The model under review builds one solid part; all positions refer to its coordinate system, in mm. Face numbers are marked on the shaded views. A direction names the side the tool comes from. Give positions to 0.01 mm unless a question says otherwise; leave off trailing zeros. Order: outer loops, then holes, each group sorted by start corner. A loop starts at its lowest first (then second) coordinate and runs counter-clockwise, first axis right, second up. Notation, with made-up numbers: (13.5, 31) -> (52.5, 31) arc R20 cw to (52.5, 35) -> close; hole circle Ø5 at (32, 71). An arc over 180 degrees is marked (long way). Answer as a JSON object with one key per item and string values. Group by question number.
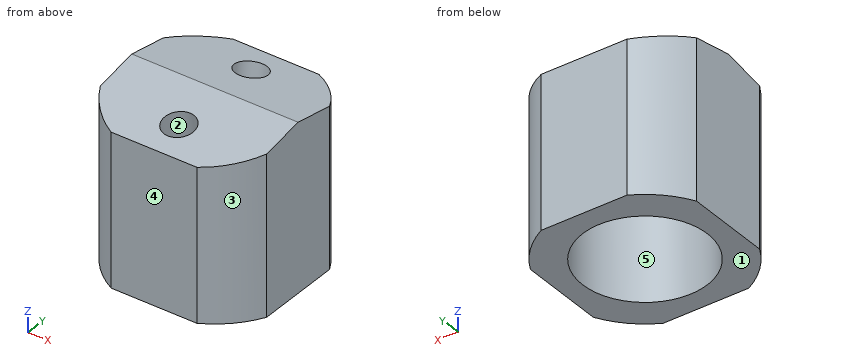
from build123d import *

# Parameters (mm, degrees)
F0_W     = 101.6
F0_H     = 101.6
F1_DEPTH = 50.8
F2_R     = 38.1
F3_DEPTH = 76.2
F5_DEPTH = 50.8
F6_R     = 9.525
F7_DEPTH = 25.4
F9_DEPTH = 127


# Not quite as in the source:
# - a pattern or mirror of a feature is missing from the dataset's text; its kind, count and spacing are read off the source's solid


with BuildPart() as f1:
    # F0 (on Top) → F1 (new body, symmetric)
    with BuildSketch(Plane.XY):
        Rectangle(F0_W, F0_H)
    extrude(amount=F1_DEPTH, both=True)

    # F2 (on face) → F3 (cut)
    with BuildSketch(Plane(origin=(0, 0, -50.8), x_dir=(1, 0, 0), z_dir=(0, 0, -1))):
        Circle(F2_R)
    extrude(amount=-F3_DEPTH, mode=Mode.SUBTRACT)

    # F4 (on Right) → F5 (cut, symmetric)
    with BuildSketch(Plane.YZ):
        Polygon((-50.8, 41.84258938), (0, 50.8), (-50.8, 50.8), align=None)
    f5 = extrude(amount=F5_DEPTH, both=True, mode=Mode.SUBTRACT)

    # F5_copies: F5 across plane
    add(f5.mirror(Plane.ZX), mode=Mode.SUBTRACT)

    # F6 (on face) → F7 (cut)
    with BuildSketch(Plane(origin=(0, -8.6873116405, 49.268192568), x_dir=(1, 0, 0), z_dir=(0, -0.1736481777, 0.984807753))):
        with Locations((0, -21.6586725745)):
            Circle(F6_R)
    f7 = extrude(amount=-F7_DEPTH, mode=Mode.SUBTRACT)

    # F7_copies: F7 across plane
    add(f7.mirror(Plane.ZX.offset(5e-06)), mode=Mode.SUBTRACT)

    # F8 (on face) → F9 (cut)
    with BuildSketch(Plane(origin=(0, 0, -50.8), x_dir=(1, 0, 0), z_dir=(0, 0, -1))):
        with BuildLine():
            ThreePointArc((26.1817207227, 50.8), (40.4111525448, 40.4111525448), (50.8, 26.1817207227))
            Line((50.8, 26.1817207227), (50.8, 50.8))
            Line((50.8, 50.8), (26.1817207227, 50.8))
        make_face()
        with BuildLine():
            Line((50.8, -50.8), (50.8, -26.1817207227))
            ThreePointArc((50.8, -26.1817207227), (40.4111525448, -40.4111525448), (26.1817207227, -50.8))
            Line((26.1817207227, -50.8), (50.8, -50.8))
        make_face()
        with BuildLine():
            Line((-26.1817207227, 50.8), (26.1817207227, 50.8))
            ThreePointArc((26.1817207227, 50.8), (0, 57.15), (-26.1817207227, 50.8))
        make_face()
        with BuildLine():
            ThreePointArc((-50.8, 26.1817207227), (-40.4111525448, 40.4111525448), (-26.1817207227, 50.8))
            Line((-26.1817207227, 50.8), (-50.8, 50.8))
            Line((-50.8, 50.8), (-50.8, 26.1817207227))
        make_face()
        with BuildLine():
            Line((-50.8, -50.8), (-26.1817207227, -50.8))
            ThreePointArc((-26.1817207227, -50.8), (-40.4111525448, -40.4111525448), (-50.8, -26.1817207227))
            Line((-50.8, -26.1817207227), (-50.8, -50.8))
        make_face()
    extrude(amount=-F9_DEPTH, mode=Mode.SUBTRACT)


solid = f1.part
1. Machinability: for the marked faces 4 and 5, which of the approach directions +Z, -Z, +X, -X, +Y, -Y give a long, thin tool a straight path to every point of the face, cutting with its end or side? Answer none if there is none.
2. Take a section at C-C on y = 2. Give the boundary of the cut face in (x, z), plus the area to 3 significant figures.
3. For pin 1 (8 mm diameter, centred on x = -17.5, y = -38.5, fed in from +Z); pin 2 (1 mm diameter, centred on x = -24.5, y = -1.5, fed in from +Z); pin 3 (1 mm diameter, centred on x = 26.5, y = -7, fed in from -Z), all flat-tipped, find the tip position at first contact; note any pin that passes through.
4. Draft analysis for pull direction Y (two halves, no side actions). For the marked faces 1, 2 and 3, state which applies: pulls with the +Y half, pulls with the -Y half, needs draft (parallel to the pull), parting line crosses it, or undercut.
5. Take a section at B-B on z = -23. Give the boundary of the cut face in (x, y), plus the area to 3 significant figures.
6. For probe 1 along X at (y, z) = (0, -9); probe 2 along Y at (x, z) = (14, -41), list the stretches that pass through material, from the lowest coordinate up. Write a range as [from, to].
7. Take a section at A-A on x = 0. Give the boundary of the cut face in (y, z), plus the area to 3 significant figures.
8. Take a section at D-D on x = -30. Give the boundary of the cut face in (y, z).
Checks:
{
 "1": {"face 4": "+Z, -Z, +X, -X, -Y", "face 5": "-Z"},
 "2": {"outline": "(-50.8, -50.8) -> (-38.05, -50.8) -> (-38.05, 25.4) -> (38.05, 25.4) -> (38.05, -50.8) -> (50.8, -50.8) -> (50.8, 50.45) -> (-50.8, 50.45) -> close", "area": "4,490 mm2"},
 "3": {"pin 1": "stops at z = 44.72", "pin 2": "stops at z = 50.62", "pin 3": "stops at z = 25.4"},
 "4": {"face 1": "needs draft", "face 2": "undercut", "face 3": "pulls with the -Y half"},
 "5": {"outline": "(-50.8, -26.18) arc R57.15 ccw to (-26.18, -50.8) -> (26.18, -50.8) arc R57.15 ccw to (50.8, -26.18) -> (50.8, 26.18) arc R57.15 ccw to (26.18, 50.8) -> (-26.18, 50.8) arc R57.15 ccw to (-50.8, 26.18) -> close; hole circle Ø76.2 at (0, 0)", "area": "4,800 mm2"},
 "6": {"probe 1": "x = [-50.8, -38.1], [38.1, 50.8]", "probe 2": "y = [-50.8, -35.43], [35.43, 50.8]"},
 "7": {"outline": "(-50.8, -50.8) -> (-38.1, -50.8) -> (-38.1, 25.4) -> (-36.14, 25.4) -> (-39.4, 43.85) -> (-50.8, 41.84) -> close; (-20.64, 47.16) -> (-16.8, 25.4) -> (16.8, 25.4) -> (20.64, 47.16) -> (0, 50.8) -> close; (36.14, 25.4) -> (38.1, 25.4) -> (38.1, -50.8) -> (50.8, -50.8) -> (50.8, 41.84) -> (39.4, 43.85) -> close", "area": "3,280 mm2"},
 "8": {"outline": "(-48.64, -50.8) -> (-23.49, -50.8) -> (-23.49, 25.4) -> (23.49, 25.4) -> (23.49, -50.8) -> (48.64, -50.8) -> (48.64, 42.22) -> (0, 50.8) -> (-48.64, 42.22) -> close"}
}
